Could you check a few things on this model? Use its own coordinates, in mm. Give positions to 0.01 mm unless a question says otherwise; leave off trailing zeros. Order: outer loops, then holes, each group sorted by start corner. A loop starts at its lowest first (then second) coordinate and runs counter-clockwise, first axis right, second up. Notation, with made-up numbers: (-0.5, 50.25) - (21.5, 50.25) arc R20 cw to (21.5, 87.25) - close; hole circle Ø10 at (-12.75, 52.25). An arc over 180 degrees is marked (long way). One line per question, with ' | ' between items. Start each with the question number.
1. Imagine slicing it at C-C (z = 11). Please give me the cut outline in (x, y), and give its area (3 significant figures).
2. Imagine slicing it at A-A (x = -47). Please give me the cut outline in (y, z), and give its area (3 significant figures).
3. For P1, Ø4, axis at y = -139, z = 19, coming from the -X side; P2, Ø8, axis at x = -335.41, y = -429.86, coming from the -Z side; P3, Ø6, axis at y = -149, z = 3, coming from the +X side; P4, Ø5, axis at y = -196, z = 9, coming from the +X side, each with a flat end and sliding along its axis, tell me the tip position at first contact or that it passes through.
4. Imagine slicing it at D-D (x = -236). Please give me the cut outline in (y, z).
5. I need wall thicknesses on probe 1 along Y at (x, z) = (-428, 2); probe 2 along Y at (x, z) = (-355, 4.25); probe 3 along Y at (x, z) = (-333.5, 5.75). Which ranges of each line are inside material? Lowest first, please. Write a range as from..to.
6. Imagine slicing it at B-B (y = -585.5). Please give me the cut outline in (x, z), and give its area (3 significant figures).
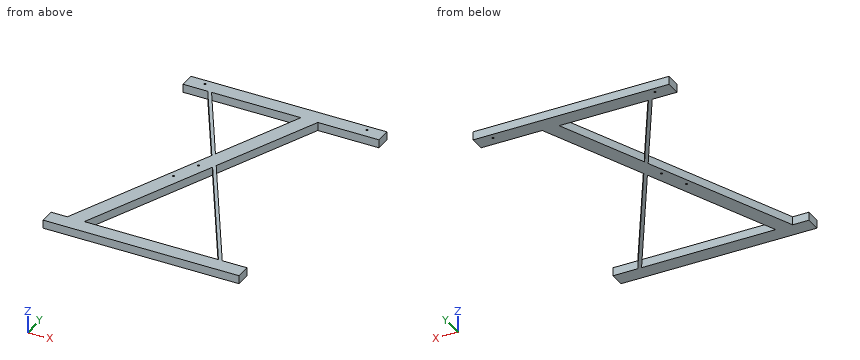
Autodesk Inventor part; units mm, degrees
ref_plane "YZ Plane" through (0, 0, 0) normal (1, 0, 0) x (0, 1, 0)
ref_plane "XZ Plane" through (0, 0, 0) normal (0, 1, 0) x (-1, 0, 0)
ref_plane "XY Plane" through (0, 0, 0) normal (0, 0, 1) x (1, 0, 0)
sketch "草图1" plane through (0, 0, 0) normal (0, 0, 1) x (1, 0, 0)
  line L0 (-510.4235, -20.2532) -> (9.5765, -20.2532)
  line L1 (9.5765, -20.2532) -> (9.5765, -60.2532)
  line L2 (9.5765, -60.2532) -> (-510.4235, -60.2532)
  line L3 (-510.4235, -60.2532) -> (-510.4235, -20.2532)
  line L4 (-510.4235, -707.2532) -> (9.5765, -707.2532)
  line L5 (9.5765, -707.2532) -> (9.5765, -747.2532)
  line L6 (9.5765, -747.2532) -> (-510.4235, -747.2532)
  line L7 (-510.4235, -747.2532) -> (-510.4235, -707.2532)
  line L8 (-66.4235, -707.2532) -> (-274.0901, -351.8026)
  line L9 (-56.4235, -707.2532) -> (-269.9235, -341.818)
  line L10 (-296.1735, -296.8875) -> (-434.4235, -60.2532)
  line L11 (-300.3401, -306.872) -> (-444.4235, -60.2532)
  line L12 (-152.4235, -60.2532) -> (-269.9235, -341.818)
  line L13 (-274.0901, -351.8026) -> (-422.4235, -707.2532)
  line L14 (-467.4235, -707.2532) -> (-300.3401, -306.872)
  line L15 (-296.1735, -296.8875) -> (-197.4235, -60.2532)
  point P0 (0, 0)
  dimension "d0" = 520
  dimension "d1" = 40
  dimension "d2" = 162
  dimension "d3" = 45
  dimension "d4" = 647
  dimension "d5" = 40
  dimension "d6" = 43
  dimension "d7" = 66
  dimension "d8" = 66
  dimension "d9" = 10
extrude "拉伸1" add sketch "草图1" along normal blind 22 contours L0 L1 L2 L3 | L2 L10 L15 L12 L9 L4 L8 L13 L14 L11 | L4 L5 L6 L7
sketch "草图2" plane through (0, 0, 22) normal (0, 0, 1) x (1, 0, 0)
  line L0 (9.5765, -60.2532) -> (9.5765, -20.2532)
  circle A0 centre (-35.4235, -35.2532) radius 2.5
  line L1 (9.5765, -20.2532) -> (-510.4235, -20.2532)
  line L2 (-510.4235, -20.2532) -> (-510.4235, -60.2532)
  circle A1 centre (-465.4235, -35.2532) radius 2.5
  line L3 (-300.3401, -306.872) -> (-467.4235, -707.2532)
  circle A2 centre (-306.5264, -360.6449) radius 2.5
  circle A3 centre (-335.4105, -429.8598) radius 2.5
  point P0 (0, 0)
  dimension "d12" = 45
  dimension "d13" = 5
  dimension "d14" = 15
  dimension "d15" = 45
  dimension "d16" = 15
  dimension "d17" = 5
  dimension "d46" = 5
  dimension "d47" = 5
  dimension "d48" = 75
extrude "拉伸2" cut sketch "草图2" against normal blind 25
thread "螺纹1"
thread "螺纹2"
properties part number "Desk stand"
Results found:
1) outline: (-510.42, -747.25) - (9.58, -747.25) - (9.58, -707.25) - (-56.42, -707.25) - (-269.92, -341.82) - (-152.42, -60.25) - (9.58, -60.25) - (9.58, -20.25) - (-510.42, -20.25) - (-510.42, -60.25) - (-444.42, -60.25) - (-300.34, -306.87) - (-467.42, -707.25) - (-510.42, -707.25) - close; hole circle Ø5 at (-465.42, -35.25); hole (-434.42, -60.25) - (-296.17, -296.89) - (-197.42, -60.25) - close; hole (-422.42, -707.25) - (-66.42, -707.25) - (-274.09, -351.8) - close; hole circle Ø5 at (-335.41, -429.86); hole circle Ø5 at (-306.53, -360.64); hole circle Ø5 at (-35.42, -35.25) | area: 76,700 mm2
2) outline: (-747.25, 0) - (-707.25, 0) - (-707.25, 22) - (-747.25, 22) - close; (-60.25, 0) - (-20.25, 0) - (-20.25, 22) - (-60.25, 22) - close | area: 1,760 mm2
3) P1: stops at x = -399.59 | P2: stops at z = 0 | P3: stops at x = -188.21 | P4: stops at x = -208.03
4) outline: (-747.25, 0) - (-707.25, 0) - (-707.25, 22) - (-747.25, 22) - close; (-417, 0) - (-399.88, 0) - (-399.88, 22) - (-417, 22) - close; (-260.53, 0) - (-152.69, 0) - (-152.69, 22) - (-260.53, 22) - close; (-60.25, 0) - (-20.25, 0) - (-20.25, 22) - (-60.25, 22) - close
5) probe 1: y = -747.25..-612.78, -88.36..-71.25, -60.25..-20.25 | probe 2: y = -747.25..-707.25, -545.69..-437.85, -213.31..-196.2, -60.25..-20.25 | probe 3: y = -747.25..-707.25, -494.17..-431.47, -428.25..-386.33, -250.11..-233, -60.25..-20.25
6) outline: (-416.61, 0) - (-371.61, 0) - (-371.61, 22) - (-416.61, 22) - close; (-137.56, 0) - (-127.56, 0) - (-127.56, 22) - (-137.56, 22) - close | area: 1,210 mm2
